Part model, mm, in its own coordinate system. Face numbers are marked on the shaded views. A direction names the side the tool comes from. Round coordinates to 2 decimals unless told otherwise and drop trailing zeros. Order: outer loops, then holes, each group sorted by start corner. A loop starts at its lowest first (then second) coordinate and runs counter-clockwise, first axis right, second up. Notation, with made-up numbers: M 25.5,49.25 L 75.5,49.25 A20 cw 75.5,64.25 Z; hole C 42,-34 d6. An arc over 180 degrees is marked long. One line per question, with ' | ' between items.
from build123d import *

# Parameters (mm, degrees)
SKETCH_R           = 14
PAD_DEPTH          = 13
SKETCH001_R        = 11.1
POCKET_DEPTH       = 13.001
SKETCH002_W        = 17
SKETCH002_H        = 4
PAD001_DEPTH       = 10
POLARPATTERN_COUNT = 2
SKETCH005_R        = 11.1
POCKET003_DEPTH    = 30.201
SKETCH006_W        = 1
SKETCH006_H        = 9.58917
POCKET004_DEPTH    = 30


with BuildPart() as part:
    # Sketch → Pad (new body)
    with BuildSketch(Plane.XY):
        Circle(SKETCH_R)
    extrude(amount=PAD_DEPTH)

    # Sketch001 → Pocket (cut, through all)
    with BuildSketch(Plane.XY.offset(13)):
        Circle(SKETCH001_R)
    extrude(amount=-POCKET_DEPTH, mode=Mode.SUBTRACT)

    # Sketch002 → Pad001 (new body)
    with BuildSketch(Plane.XY.offset(13)):
        with Locations((0, 13.1)):
            Rectangle(SKETCH002_W, SKETCH002_H)
    pad001 = extrude(amount=-PAD001_DEPTH)

    # PolarPattern: Pad001 ×2 about axis
    polarpattern_axis = Axis((0, 0, 13), (0, 0, 1))
    for i in range(1, POLARPATTERN_COUNT):
        add(pad001.rotate(polarpattern_axis, i * 360 / POLARPATTERN_COUNT))

    # Sketch005 → Pocket003 (cut, through all)
    with BuildSketch(Plane.XZ.offset(15.1)):
        with Locations((0, 19)):
            Circle(SKETCH005_R)
    extrude(amount=-POCKET003_DEPTH, mode=Mode.SUBTRACT)

    # Sketch006 → Pocket004 (cut)
    with BuildSketch(Plane.XZ.offset(15.1)):
        with Locations((0, 4.794585)):
            Rectangle(SKETCH006_W, SKETCH006_H)
    extrude(amount=-POCKET004_DEPTH, mode=Mode.SUBTRACT)


solid = part.part
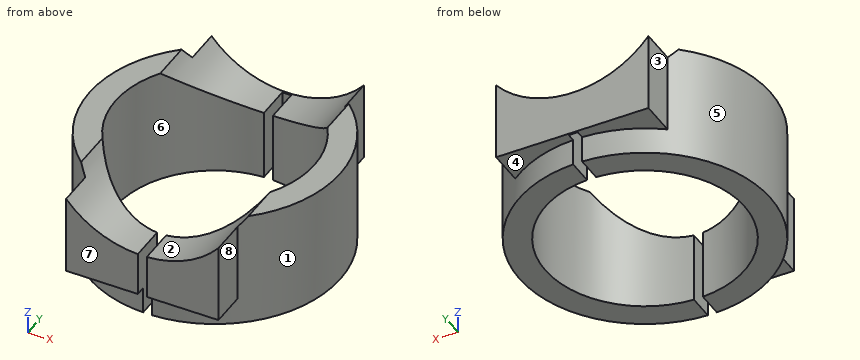
1) Saw through at B-B (x = 5.75). List the corners of the cut face in (y, z), plus the area to 3 significant figures.
The answers:
outline: M -15.1,3 L -12.76,3 L -12.76,0 L -9.49,0 L -9.49,9.51 L -15.1,9.51 Z; M 9.49,0 L 12.76,0 L 12.76,3 L 15.1,3 L 15.1,9.51 L 9.49,9.51 Z | area: 92.6 mm²
2) Saw through at C-C (y = 0). List the corners of the cut face in (x, z).
The answers:
outline: M -14,0 L -11.1,0 L -11.1,13 L -14,13 Z; M 11.1,0 L 14,0 L 14,13 L 11.1,13 Z
3) Which spindle directions (+Z, -Z, +X, -X, +Y, -Y) get a long thin tool onto all of the face, cutting with end or side? Do the marked faces 1, 2, 3 and 4. Say none if no direction does.
The answers:
face 1: -Z, +X | face 2: +Z, +Y, -Y | face 3: +Z, -Z, -X, +Y | face 4: -Z, +Y
4) Two-plate mould, pull along X, no slides. Class the marked faces 5, 6, 7 and 8: released by +X, released by -X, zero draft, split by the parting line, or undercut.
The answers:
face 5: released by -X | face 6: undercut | face 7: zero draft | face 8: released by +X
5) Probe line 1 (X direction, y = -11.5, z = 4.25); line 2 (X direction, y = 5, z = 5); line 3 (Y direction, x = -7.5, z = 3.5). List the from-to ranges inside material, lowest first. Write a range as [from, to].
The answers:
line 1: x = [-8.5, -0.5], [0.5, 8.5] | line 2: x = [-13.08, -9.91], [9.91, 13.08] | line 3: y = [-15.1, -8.18], [8.18, 15.1]
6) Saw through at D-D (y = -10). List the corners of the cut face in (x, z).
The answers:
outline: M -9.8,0 L -4.82,0 L -4.82,9 A11.1 cw -9.34,13 L -9.8,13 Z; M 4.82,0 L 9.8,0 L 9.8,13 L 9.34,13 A11.1 cw 4.82,9 Z
7) Saw through at A-A (z = 8.5). List the corners of the cut face in (x, y), plus the area to 3 significant figures.
The answers:
outline: M -8.5,-15.1 L -3.6,-15.1 L -3.6,-10.5 A11.1 cw -3.6,10.5 L -3.6,15.1 L -8.5,15.1 L -8.5,11.12 A14 ccw -8.5,-11.12 Z; M 3.6,-15.1 L 8.5,-15.1 L 8.5,-11.12 A14 ccw 8.5,11.12 L 8.5,15.1 L 3.6,15.1 L 3.6,10.5 A11.1 cw 3.6,-10.5 Z | area: 237 mm²
8) Drop flat-ended pins along their axis: pin 1 (1.5 mm diameter, centred on y = 4.5, z = 2, fed in from +X); pin 2 (2 mm diameter, centred on y = -14, z = 7.5, fed in from -X); pin 3 (1.9 mm diameter, centred on y = 12.5, z = 3, fed in from +X). Give the stop position or say it passes through.
The answers:
pin 1: stops at x = 13.49 | pin 2: stops at x = -8.5 | pin 3: stops at x = 8.5
